```python
from build123d import *

# Parameters (mm, degrees)
F0_W      = 137.506828
F0_H      = 133.092508
F1_DEPTH  = 17.5
F2_T      = -5
F3_R      = 7.5
F4_W      = 25
F4_H      = 25
F5_DEPTH  = 20
F6_W      = 25
F6_H      = 25
F7_DEPTH  = 20
F8_W      = 25
F8_H      = 25
F9_DEPTH  = 20
F10_W     = 25
F10_H     = 25
F11_DEPTH = 20
F12_R     = 3.5
F13_DEPTH = 68
F14_R     = 3.5
F15_DEPTH = 68


with BuildPart() as f1:
    # F0 (on Front) → F1 (new body, symmetric)
    with BuildSketch(Plane.XZ):
        Rectangle(F0_W, F0_H)
    extrude(amount=F1_DEPTH, both=True)

    # F2
    f2_openings = [f1.faces().sort_by_distance(p)[0] for p in [
        (0, 17.5, 0),
    ]]
    offset(amount=F2_T, openings=f2_openings)

    # F3
    f3_edges = [f1.edges().sort_by_distance(p)[0] for p in [
        (0, -17.5, -66.546254),
        (68.753414, -17.5, 0),
        (0, -17.5, 66.546254),
        (-68.753414, -17.5, 0),
    ]]
    fillet(f3_edges, radius=F3_R)

    # F4 (on face) → F5 (join)
    with BuildSketch(Plane.XZ.offset(17.5)):
        with Locations((-48.753414, 46.546254)):
            Rectangle(F4_W, F4_H)
    extrude(amount=F5_DEPTH)

    # F6 (on face) → F7 (join)
    with BuildSketch(Plane.XZ.offset(17.5)):
        with Locations((48.753414, 46.546254)):
            Rectangle(F6_W, F6_H)
    extrude(amount=F7_DEPTH)

    # F8 (on face) → F9 (join)
    with BuildSketch(Plane.XZ.offset(17.5)):
        with Locations((-48.753414, -46.546254)):
            Rectangle(F8_W, F8_H)
    extrude(amount=F9_DEPTH)

    # F10 (on face) → F11 (join)
    with BuildSketch(Plane.XZ.offset(17.5)):
        with Locations((48.753414, -46.546254)):
            Rectangle(F10_W, F10_H)
    extrude(amount=F11_DEPTH)

    # F12 (on face) → F13 (join)
    with BuildSketch(Plane(origin=(0, 0, 34.046254), x_dir=(1, 0, 0), z_dir=(0, 0, -1))):
        with Locations((-48.423063, 25.617592)):
            Circle(F12_R)
    extrude(amount=F13_DEPTH)

    # F14 (on face) → F15 (join)
    with BuildSketch(Plane(origin=(0, 0, 34.046254), x_dir=(1, 0, 0), z_dir=(0, 0, -1))):
        with Locations((48.201937, 25.032593)):
            Circle(F14_R)
    extrude(amount=F15_DEPTH)


solid = f1.part
```
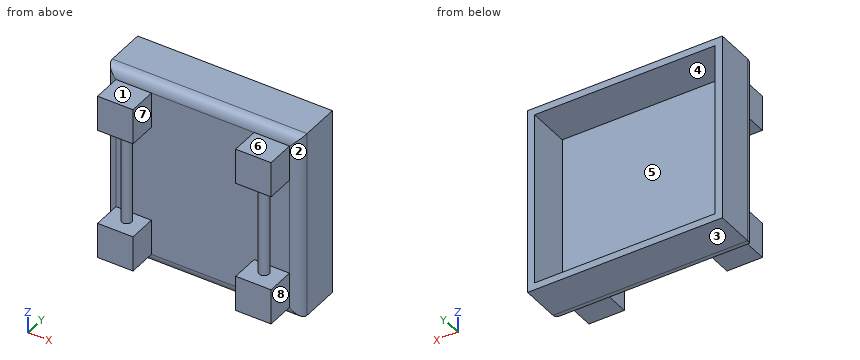
Input: part model. Units: mm. Frame: model coordinates. Face numbers are marked on the shaded views. A direction names the side the tool comes from. Coordinates: 2 decimals unless noted, no trailing zeros. Write each loop counter-clockwise with the first axis right and the second up, starting at its lowest first coordinate (ties: lowest second). Pieces come first, ordered by that corner, then holes.
1) Section C-C on y = -31.5. Output: boundary loops of the cut face in (x, z).
2) Section D-D on z = -17. Output: boundary loops of the cut face in (x, y), and give its area (3 significant figures).
3) Pin query (flat end, axial travel): pin 1 Ø6 at (y, z) = (-31.5, -44) entering from -X; pin 2 Ø6 at (x, z) = (25.5, -27) entering from +Y; pin 3 Ø10 at (x, y) = (42.5, -26) entering from -Z; pin 4 Ø6 at (x, y) = (-4.5, -12) entering from -Z. Return the tip coordinate at first contact, or that it passes through.
4) Section A-A on y = 2. Output: boundary loops of the cut face in (x, z).
5) Material intervals for line 1 along Z through (x, y) = (-8, 10); line 2 along X through (y, z) = (-9, -42.5); line 3 along Z through (x, y) = (43.5, -23.5), sorted ascending.
6) Set-up query: the marked faces 5, 6, 7 and 8. Return all of +Z, -Z, +X, -X, +Y, -Y with unobstructed straight access to the full face (end or side cutting, diameter ignored); none if empty.
7) Mould query, pull axis Z, two halves, no side actions, for the marked faces 1, 2, 3 and 4. Classes: pulls with the +Z half, pulls with the -Z half, needs draft (parallel to the pull), parting line crosses it, or undercut.
8) Section B-B on x = 29. Output: boundary loops of the cut face in (y, z), and give its area (3 significant figures).
Check result:
1. outline: (-61.25, -59.05) - (-36.25, -59.05) - (-36.25, -34.05) - (-61.25, -34.05) - close; (-61.25, 34.05) - (-36.25, 34.05) - (-36.25, 59.05) - (-61.25, 59.05) - close; (36.25, -59.05) - (61.25, -59.05) - (61.25, -34.05) - (36.25, -34.05) - close; (36.25, 34.05) - (61.25, 34.05) - (61.25, 59.05) - (36.25, 59.05) - close
2. outline: (-68.75, -10) arc R7.5 ccw to (-61.25, -17.5) - (61.25, -17.5) arc R7.5 ccw to (68.75, -10) - (68.75, 17.5) - (63.75, 17.5) - (63.75, -12.5) - (-63.75, -12.5) - (-63.75, 17.5) - (-68.75, 17.5) - close; circle Ø7 at (-48.42, -25.62); circle Ø7 at (48.2, -25.03)
2. area: 1,040 mm2
3. pin 1: stops at x = -61.25
3. pin 2: stops at y = -12.5
3. pin 3: stops at z = -59.05
3. pin 4: stops at z = -66.55
4. outline: (-68.75, -66.55) - (68.75, -66.55) - (68.75, 66.55) - (-68.75, 66.55) - close; hole (-63.75, -61.55) - (63.75, -61.55) - (63.75, 61.55) - (-63.75, 61.55) - close
5. line 1: z = -66.55 to -61.55, 61.55 to 66.55
5. line 2: x = -68.75 to -63.75, 63.75 to 68.75
5. line 3: z = -59.05 to -34.05, 34.05 to 59.05
6. face 5: +Y
6. face 6: +Z, +X, -X, -Y
6. face 7: +Z, -Z, -Y
6. face 8: +Z, -Z, +X, -Y
7. face 1: pulls with the +Z half
7. face 2: needs draft
7. face 3: pulls with the -Z half
7. face 4: undercut
8. outline: (-17.5, -59.05) arc R7.5 ccw to (-10, -66.55) - (17.5, -66.55) - (17.5, -61.55) - (-12.5, -61.55) - (-12.5, 61.55) - (17.5, 61.55) - (17.5, 66.55) - (-10, 66.55) arc R7.5 ccw to (-17.5, 59.05) - close
8. area: 941 mm2
